```python
from build123d import *

# Parameters (mm, degrees)
F0_W     = 40.4
F0_H     = 40.4
F1_DEPTH = 1
F3_D     = 3.3


with BuildPart() as f1:
    # F0 (on Front) → F1 (new body)
    with BuildSketch(Plane.XZ):
        with Locations((20.2, 20.2)):
            Rectangle(F0_W, F0_H)
    extrude(amount=F1_DEPTH)

    # F3 (through all)
    with Locations(Plane.XZ.offset(1)):
        with Locations((4.2, 36.2), (36.2, 36.2), (36.2, 4.2), (4.2, 4.2)):
            Hole(F3_D / 2)


solid = f1.part
```
For this review, take the finished solid that the model builds, in its own axes (mm). Give positions to 0.01 mm unless a question says otherwise; leave off trailing zeros. Write each loop counter-clockwise with the first axis right and the second up, starting at its lowest first coordinate (ties: lowest second). Pieces come first, ordered by that corner, then holes.
Item 1: Take a section at B-B (y = -0.6). Give the boundary of the cut face in (x, z).
Item 2: Insertion check: P1, Ø4, axis at x = 4.2, z = 4.2, coming from the -Y side; P2, Ø2.5, axis at x = 36.2, z = 36.2, coming from the +Y side. Each pin has a flat end and moves straight along its axis. Give the tip position at first contact, or say it passes through.
Item 3: The part is to be moulded in two halves that separate along Z. For faces 1 (the face through (19.9, -0.5, 40.4)), 2 (the face through (20, -1, 20)), 3 (the face through (4.415, -0.493, 5.836)), say which applies: +Z half, -Z half, draft (parallel to the pull), parting line (faces both ways), or undercut.
Item 4: Wall thickness on probe 1 along Z at (x, y) = (4.2, -0.3); probe 2 along Z at (x, y) = (35, -0.4); probe 3 along X at (y, z) = (-0.1, 36.5): over which ranges is each line inside the solid? List them lowest first.
Item 5: Take a section at A-A (z = 4.2). Give the boundary of the cut face in (x, y).
Item 6: Take a section at C-C (x = 4.2). Give the boundary of the cut face in (y, z).
Established:
1. outline: (0, 0) - (40.4, 0) - (40.4, 40.4) - (0, 40.4) - close; hole circle Ø3.3 at (4.2, 4.2); hole circle Ø3.3 at (4.2, 36.2); hole circle Ø3.3 at (36.2, 4.2); hole circle Ø3.3 at (36.2, 36.2)
2. P1: stops at y = -1
2. P2: passes through
3. face 1: +Z half
3. face 2: draft
3. face 3: undercut
4. probe 1: z = 0 to 2.55, 5.85 to 34.55, 37.85 to 40.4
4. probe 2: z = 0 to 3.07, 5.33 to 35.07, 37.33 to 40.4
4. probe 3: x = 0 to 2.58, 5.82 to 34.58, 37.82 to 40.4
5. outline: (0, -1) - (2.55, -1) - (2.55, 0) - (0, 0) - close; (5.85, -1) - (34.55, -1) - (34.55, 0) - (5.85, 0) - close; (37.85, -1) - (40.4, -1) - (40.4, 0) - (37.85, 0) - close
6. outline: (-1, 0) - (0, 0) - (0, 2.55) - (-1, 2.55) - close; (-1, 5.85) - (0, 5.85) - (0, 34.55) - (-1, 34.55) - close; (-1, 37.85) - (0, 37.85) - (0, 40.4) - (-1, 40.4) - close
